The drawing under review shows one solid part. Ordinate dimensions are in mm from its lowest x, y, z. Coordinates: 2 decimals unless noted, no trailing zeros. Order: outer loops, then holes, each group sorted by start corner. A loop starts at its lowest first (then second) coordinate and runs counter-clockwise, first axis right, second up.
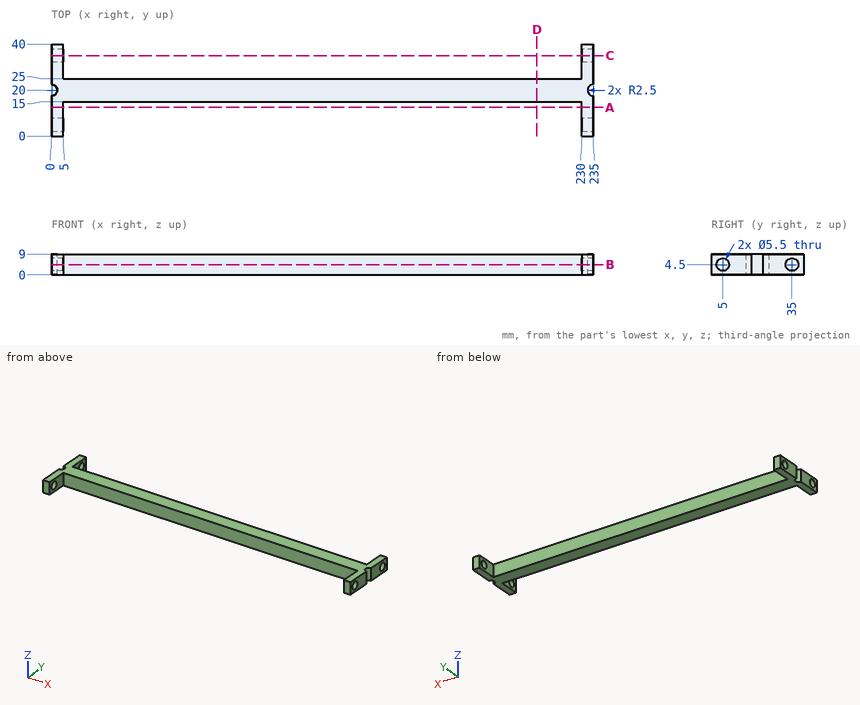
(1) Wall thickness on probe 1 along Z at (x, y) = (2.5, 35); probe 2 along X at (y, z) = (37, 7.5); probe 3 along Y at (x, z) = (86.5, 5): over which ranges is each line inside the solid? List them lowest first.
A:
probe 1: z = 0 to 1.75, 7.25 to 9
probe 2: x = 0 to 5, 230 to 235
probe 3: y = 15 to 25
(2) We need section A-A, the plane y = 12.5. Write out the cut boundary in (x, z).
A:
outline: (0, 0) - (5, 0) - (5, 9) - (0, 9) - close; (230, 0) - (235, 0) - (235, 9) - (230, 9) - close
(3) We need section B-B, the plane z = 4.5. Count the separate pieces of the cut face and the enclosed holes in it, and give its area (3 significant figures).
A:
separate pieces: 5
enclosed holes: 0
area: 2,520 mm2
(4) We need section C-C, the plane y = 35. Write out the cut boundary in (x, z).
A:
outline: (0, 0) - (5, 0) - (5, 1.75) - (0, 1.75) - close; (0, 7.25) - (5, 7.25) - (5, 9) - (0, 9) - close; (230, 0) - (235, 0) - (235, 1.75) - (230, 1.75) - close; (230, 7.25) - (235, 7.25) - (235, 9) - (230, 9) - close
(5) For pin 1 Ø1 at (x, z) = (72, 5) entering from +Y; pin 2 Ø1 at (x, z) = (86.5, 7.5) entering from -Y, all flat-tipped, find the tip position at first contact; note any pin that passes through.
A:
pin 1: stops at y = 25
pin 2: stops at y = 15
(6) We need section D-D, the plane x = 210.5. Write out the cut boundary in (y, z), and give its area (3 significant figures).
A:
outline: (15, 0) - (25, 0) - (25, 9) - (15, 9) - close
area: 90.0 mm2
